Input: part model. Units: mm. Frame: model coordinates. A direction names the side the tool comes from. Round coordinates to 2 decimals unless told otherwise and drop trailing zeros. Order: outer loops, then holes, each group sorted by start corner. A loop starts at its lowest first (then second) coordinate and runs counter-clockwise, first axis right, second up. Notation, with made-up numbers: M 41,9 L 58,9 A21 ccw 58,26 Z; hole C 4,83 d4. An arc over 180 degrees is marked long. One line per question, with ' | ' between items.
```python
from build123d import *
from build123d.topology import SkipClean

# Parameters (mm, degrees)
SKETCH_1_R          = 25
EXTRUDE_2_DEPTH     = 2
EXTRUDE_3_DEPTH     = 45
SKETCH_3_R          = 21.5
SKETCH_3_R_2        = 20.5
EXTRUDE_4_DEPTH     = 45
SKETCH_5_R          = 21.5
EXTRUDE_5_DEPTH     = 16
CUT_EXTRUDE_1_DEPTH = 16


with BuildPart() as part:
    # 草图1 → 凸台-拉伸2 (new body)
    with BuildSketch(Plane(origin=(0, 0, 0), x_dir=(1, 0, 0), z_dir=(0, 1, 0))):
        with Locations(Location((0, 0, 0), (0, 0, 270))):
            Circle(SKETCH_1_R)
    extrude(amount=EXTRUDE_2_DEPTH)

    # 草图2 → 凸台-拉伸3 (add)
    with BuildSketch(Plane(origin=(0, 2, 0), x_dir=(1, 0, 0), z_dir=(0, 1, 0))):
        with BuildLine():
            Line((46.976057732, -1.5), (20.4450483, -1.5))
            ThreePointArc((20.4450483, -1.5), (20.5, 0), (20.4450483, 1.5))
            Line((20.4450483, 1.5), (46.976057732, 1.5))
            ThreePointArc((46.976057732, 1.5), (47, 0), (46.976057732, -1.5))
        make_face()
        with BuildLine():
            Line((8.840104317, -18.311509822), (22.189479497, -41.433305883))
            ThreePointArc((22.189479497, -41.433305883), (23.500412361, -40.704084016), (24.787406337, -39.933398601))
            Line((24.787406337, -39.933398601), (11.438034851, -16.811608937))
            ThreePointArc((11.438034851, -16.811608937), (10.166767318, -17.609533741), (8.840104317, -18.311509822))
        make_face()
        with BuildLine():
            Line((-8.923486044, -18.45593121), (-22.18899076, -41.432459365))
            ThreePointArc((-22.18899076, -41.432459365), (-23.5, -40.703193978), (-24.787066971, -39.932459365))
            Line((-24.787066971, -39.932459365), (-11.521562256, -16.95593121))
            ThreePointArc((-11.521562256, -16.95593121), (-10.25, -17.753520778), (-8.923486044, -18.45593121))
        make_face()
        with BuildLine():
            Line((-20.4450483, 1.5), (-46.976057732, 1.5))
            ThreePointArc((-46.976057732, 1.5), (-47, 0), (-46.976057732, -1.5))
            Line((-46.976057732, -1.5), (-20.4450483, -1.5))
            ThreePointArc((-20.4450483, -1.5), (-20.5, 0), (-20.4450483, 1.5))
        make_face()
        with BuildLine():
            Line((-11.521562256, 16.95593121), (-24.787066971, 39.932459365))
            ThreePointArc((-24.787066971, 39.932459365), (-23.5, 40.703193978), (-22.18899076, 41.432459365))
            Line((-22.18899076, 41.432459365), (-8.923486044, 18.45593121))
            ThreePointArc((-8.923486044, 18.45593121), (-10.25, 17.753520778), (-11.521562256, 16.95593121))
        make_face()
        with BuildLine():
            Line((8.923486044, 18.45593121), (22.18899076, 41.432459365))
            ThreePointArc((22.18899076, 41.432459365), (23.5, 40.703193978), (24.787066971, 39.932459365))
            Line((24.787066971, 39.932459365), (11.521562256, 16.95593121))
            ThreePointArc((11.521562256, 16.95593121), (10.25, 17.753520778), (8.923486044, 18.45593121))
        make_face()
    extrude(amount=EXTRUDE_3_DEPTH)

    # 草图3 → 凸台-拉伸4 (add)
    with SkipClean():  # the faces are left unmerged after this step: merging them gives an invalid solid
        with BuildSketch(Plane(origin=(0, 2, 0), x_dir=(1, 0, 0), z_dir=(0, 1, 0))):
            Circle(SKETCH_3_R)
            Circle(SKETCH_3_R_2, mode=Mode.SUBTRACT)
        extrude(amount=EXTRUDE_4_DEPTH)

    # 草图5 → 凸台-拉伸5 (add)
    with BuildSketch(Plane(origin=(0, 2, 0), x_dir=(1, 0, 0), z_dir=(0, 1, 0))):
        Circle(SKETCH_5_R)
    extrude(amount=EXTRUDE_5_DEPTH)

    # 草图6 → 切除-拉伸1 (cut)
    with BuildSketch(Plane(origin=(0, 18, 0), x_dir=(1, 0, 0), z_dir=(0, 1, 0))):
        with BuildLine():
            Line((2.1, 14.9), (2.9, 1.95))
            Line((2.9, 1.95), (8.35, 1.95))
            ThreePointArc((8.35, 1.95), (10.3, 0), (8.35, -1.95))
            Line((8.35, -1.95), (3.5, -1.95))
            Line((3.5, -1.95), (2.1, -17.9))
            ThreePointArc((2.1, -17.9), (0, -20), (-2.1, -17.9))
            Line((-2.1, -17.9), (-3.5, -1.95))
            Line((-3.5, -1.95), (-8.35, -1.95))
            ThreePointArc((-8.35, -1.95), (-10.3, 0), (-8.35, 1.95))
            Line((-8.35, 1.95), (-2.9, 1.95))
            Line((-2.9, 1.95), (-2.1, 14.9))
            ThreePointArc((-2.1, 14.9), (0, 17), (2.1, 14.9))
        make_face()
    extrude(amount=-CUT_EXTRUDE_1_DEPTH, mode=Mode.SUBTRACT)


solid = part.part
```
Item 1: Section query D-D, the plane z = -8.5. Return loops of the section in (x, y), plus the area to 3 significant figures.
Report:
outline: M -23.51,0 L 23.51,0 L 23.51,2 L 19.75,2 L 19.75,47 L 18.65,47 L 18.65,18 L 2.5,18 L 2.5,2 L -2.5,2 L -2.5,18 L -18.65,18 L -18.65,47 L -19.75,47 L -19.75,2 L -23.51,2 Z | area: 710 mm²
Item 2: Access query for faces 5 (the flat face through (18, 2, 31)), 6 (the flat face through (-6, 10, -1.95)), 7 (the cylindrical face through (18.69, 24.18, -10.63)). Directions: +Z, -Z, +X, -X, +Y, -Y. A direction counts if a zero-diameter tool reaches every point of the face in a straight line with its end or side. Return the directions, or none.
Report:
face 5: +Z, +X, -Y | face 6: +Y | face 7: +X, +Y
Item 3: Section query B-B, the plane z = -34.5. Return loops of the section in (x, y).
Report:
outline: M -21.65,2 L -18.19,2 L -18.19,47 L -21.65,47 Z; M 18.19,2 L 21.65,2 L 21.65,47 L 18.19,47 Z
Item 4: Section query A-A, the plane x = -15.5. Return loops of the section in (y, z), plus the area to 3 significant figures.
Report:
outline: M 0,-19.62 L 2,-19.62 L 2,-14.9 L 47,-14.9 L 47,-13.42 L 18,-13.42 L 18,13.42 L 47,13.42 L 47,14.9 L 2,14.9 L 2,19.62 L 0,19.62 Z; M 2,-29.85 L 47,-29.85 L 47,-23.85 L 2,-23.85 Z; M 2,23.85 L 47,23.85 L 47,29.85 L 2,29.85 Z | area: 1,180 mm²
Item 5: Mould query, pull axis Z, two halves, no side actions, for faces 1 (the cylindrical face through (-0.1, 24.2, 21.5)), 2 (the cylindrical face through (23.482, 24.185, -40.714)), 3 (the cylindrical face through (-18.69, 24.18, 10.63)), 4 (the flat face through (-18, 2, 31)). Classes: +Z half, -Z half, draft (parallel to the pull), parting line (faces both ways), or undercut.
Report:
face 1: +Z half | face 2: -Z half | face 3: undercut | face 4: draft
Item 6: Section query C-C, the plane x = 0. Return loops of the section in (y, z), plus the area to 3 significant figures.
Report:
outline: M 0,-25 L 2,-25 L 2,-21.5 L 47,-21.5 L 47,-20.5 L 18,-20.5 L 18,-17 L 2,-17 L 2,20 L 18,20 L 18,20.5 L 47,20.5 L 47,21.5 L 2,21.5 L 2,25 L 0,25 Z | area: 254 mm²
Item 7: Line query: line 1 along Z through (x, y) = (18, 27.5); line 2 along Z through (x, y) = (32.5, 12.5); line 3 along Z through (x, y) = (13.5, 3.5). Output: solid intervals per line, ascending. Write a range as from..to.
Report:
line 1: -34.18..-28.18, -11.76..-9.81, 9.81..11.76, 28.18..34.18 | line 2: -1.5..1.5 | line 3: -26.38..-20.38, -16.73..16.73, 20.38..26.38
Item 8: First-contact query: pin 1 (8 mm diameter, centred on x = -12.5, z = -23, fed in from -Y); pin 2 (4 mm diameter, centred on y = 40, z = -19, fed in from -X); pin 3 (4 mm diameter, centred on x = 19.5, y = 6, fed in from +Z); pin 4 (2.5 mm diameter, centred on x = -4.5, y = 12.5, fed in from +Z). Flat tips, straight axial feed; report the tip coordinate or a pass-through.
Report:
pin 1: y = 0 | pin 2: x = -13.86 | pin 3: z = 40.24 | pin 4: z = 21.25
